Geometry: final body of the model. Coordinates: model frame, mm. A direction names the side the tool comes from. Give positions to 0.01 mm unless a question says otherwise; leave off trailing zeros. Write each loop counter-clockwise with the first axis right and the second up, starting at its lowest first coordinate (ties: lowest second). Pieces come first, ordered by that corner, then holes. Notation, with made-up numbers: M -15,58 L 12,58 A31 ccw 12,84 Z; hole C 19,52 d6. An arc over 180 degrees is marked long. Use one line per item in the form item = value. Start each with the question number.
Item 1: Access query for faces 1 (the flat face through (2, -2.5, -2)), 2 (the cylindrical face through (0.95, -2.313, -4.338)). Directions: +Z, -Z, +X, -X, +Y, -Y. A direction counts if a zero-diameter tool reaches every point of the face in a straight line with its end or side. Return the directions, or none.
Item 2: Section query D-D on z = -5.75. Return loops of the section in (x, y), then the cut area to 3 significant figures.
Item 3: Section query C-C on z = -3.5. Return loops of the section in (x, y).
Item 4: Section query A-A on y = -2.4. Return loops of the section in (x, z).
Item 5: Section query B-B on x = 5.75. Return loops of the section in (y, z).
Item 6: Material intervals for line 1 along Z through (x, y) = (-2.5, -2.25); line 2 along Z through (x, y) = (6, -2.35); line 3 along Z through (x, y) = (5, -2.4), sorted ascending. Write a range as from..to.
from build123d import *

# Parameters (mm, degrees)
SKETCH_1_W          = 12.642384092
SKETCH_1_H          = 0.502134845
EXTRUDE_1_DEPTH     = 2
EXTRUDE_2_DEPTH     = 10.8
SKETCH_4_R          = 3
CUT_EXTRUDE_2_DEPTH = 10


with BuildPart() as part:
    # 스케치1 → 보스-돌출1 (new body)
    with BuildSketch(Plane.XY):
        with Locations((0.821192046, -2.248932578)):
            Rectangle(SKETCH_1_W, SKETCH_1_H)
    extrude(amount=EXTRUDE_1_DEPTH)

    # 스케치2 → 보스-돌출2 (add)
    with BuildSketch(Plane.XY.offset(2)):
        with BuildLine():
            Line((1.502842247, -1.997865155), (7.142384092, -1.997865155))
            Line((7.142384092, -1.997865155), (7.142384092, -2.5))
            Line((7.142384092, -2.5), (0, -2.5))
            ThreePointArc((0, -2.5), (0.79225536, -2.371145597), (1.502842247, -1.997865155))
        make_face()
    extrude(amount=-EXTRUDE_2_DEPTH)

    # 스케치4 → 컷-돌출2 (cut)
    with BuildSketch(Plane.XZ.offset(2.5)):
        with Locations((7.642384092, -3.5)):
            Circle(SKETCH_4_R)
    extrude(amount=-CUT_EXTRUDE_2_DEPTH, mode=Mode.SUBTRACT)


solid = part.part
Answer sheet:
q1.face_1 = +Z, -Z, +X, -X, -Y
q1.face_2 = -Z, -X, +Y
q2.outline = M 0,-2.5 L 5.66,-2.5 L 5.66,-2 L 1.5,-2 A2.5 cw Z
q2.area = 2.33 mm2
q3.outline = M 0,-2.5 L 4.64,-2.5 L 4.64,-2 L 1.5,-2 A2.5 cw Z
q4.outline = M -5.5,0 L 0.7,0 L 0.7,-8.8 L 7.14,-8.8 L 7.14,-6.46 A3 cw 7.14,-0.54 L 7.14,2 L -5.5,2 Z
q5.outline = M -2.5,-8.8 L -2,-8.8 L -2,-5.83 L -2.5,-5.83 Z; M -2.5,-1.17 L -2,-1.17 L -2,2 L -2.5,2 Z
q6.line_1 = 0..2
q6.line_2 = -8.8..-6.01, -0.99..2
q6.line_3 = -8.8..-4.92, -2.08..2
